from build123d import *

# Parameters (mm, degrees)
SKETCH012_R      = 2.5
PAD006_DEPTH     = 59
POCKET003_DEPTH  = 18
CHAMFER002_SIZE2 = 0.4
CHAMFER002_SIZE  = 0.8


with BuildPart() as part:
    # Sketch012 → Pad006 (new body)
    with BuildSketch(Plane.XY):
        Circle(SKETCH012_R)
    extrude(amount=PAD006_DEPTH)

    # Sketch013 (on Face3 of Pad006) → Pocket003 (cut)
    with BuildSketch(Plane.XY.offset(59)):
        with BuildLine():
            ThreePointArc((2, -1.5), (2.5, 0), (2, 1.5))
            Line((2, 1.5), (2, -1.5))
        make_face()
    extrude(amount=-POCKET003_DEPTH, mode=Mode.SUBTRACT)

    # Chamfer002
    chamfer002_edges = [part.edges().sort_by_distance(p)[0] for p in [
        (-2.5, 0, 59),
        (-2.5, 0, 0),
    ]]
    chamfer002_side = part.faces().sort_by_distance((-2.5, 0, 29.5))[0]
    chamfer(chamfer002_edges, length=CHAMFER002_SIZE, length2=CHAMFER002_SIZE2, reference=chamfer002_side)


with BuildPart() as part_1:
    # Body003 placement: moved
    add(part.part.moved(Location((0, 0, 2.8))))


solid = part_1.part
For this review, take the finished solid that the model builds, in its own axes (mm). A direction names the side the tool comes from. Give positions to 0.01 mm unless a question says otherwise; leave off trailing zeros. Loops run counter-clockwise (first coordinate to the right, second up) from the corner with the lowest first, then second, coordinate; pieces in that order, holes last.
Item 1: Insertion check: pin 1 (0.9 mm diameter, centred on y = -0.5, z = 56.5, fed in from +X); pin 2 (0.5 mm diameter, centred on x = 2.5, y = 0, fed in from +Z). Each pin has a flat end and moves straight along its axis. Give the tip position at first contact, or say it passes through.
Item 2: Tool access review of faces 1 (the flat face through (2, 0, 53)), 2 (the cylindrical face through (-2.5, 0.1, 31.9)): name each direction out of +Z, -Z, +X, -X, +Y, -Y from which nothing blocks a thin tool from reaching the whole face with its end or side.
Item 3: Take a section at C-C, the plane z = 48.5. State the section outline as (x, y) points.
Item 4: Take a section at B-B, the plane z = 8. State the section outline as (x, y) points, and give its area (3 significant figures).
Item 5: For line 1 along Y through (x, z) = (0.25, 24); line 2 along X through (y, z) = (0.15, 45); line 3 along Y through (x, z) = (-1.8, 15.5), list the stretches that pass through material, from the lowest coordinate up.
Item 6: Take a section at A-A, the plane y = 0. State the section outline as (x, z) points, and give its area (3 significant figures).
Calculated:
1. pin 1: stops at x = 2
1. pin 2: stops at z = 43.8
2. face 1: +Z, +X, +Y, -Y
2. face 2: +Z, -Z
3. outline: (2, -1.5) - (2, 1.5) arc R2.5 ccw (long way) to start
4. outline: circle Ø5 at (0, 0)
4. area: 19.6 mm2
5. line 1: y = -2.49 to 2.49
5. line 2: x = -2.5 to 2
5. line 3: y = -1.73 to 1.73
6. outline: (-2.5, 3.6) - (-2.1, 2.8) - (2.1, 2.8) - (2.5, 3.6) - (2.5, 43.8) - (2, 43.8) - (2, 61.8) - (-2.1, 61.8) - (-2.5, 61) - close
6. area: 286 mm2
